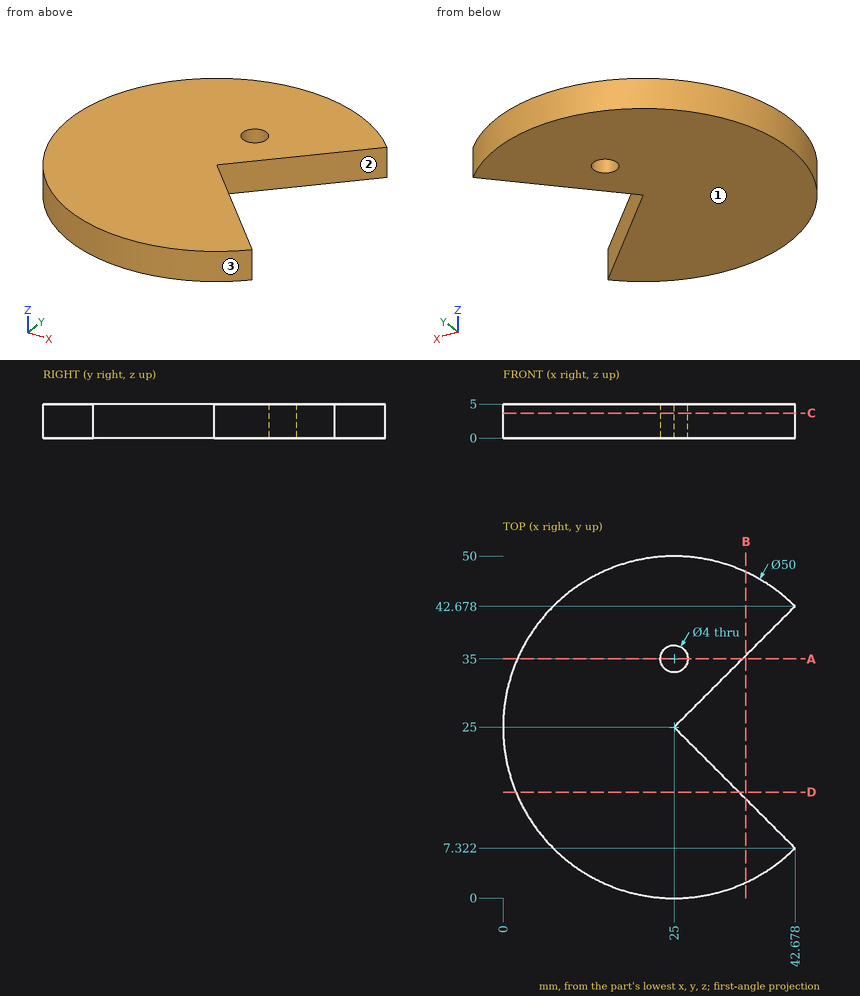
Geometry: see drawing. Coordinates: mm, zero at the bounding-box minimum. Coordinates: 2 decimals unless noted, no trailing zeros. Loops run counter-clockwise (first coordinate to the right, second up) from the corner with the lowest first, then second, coordinate; pieces in that order, holes last. Notation, with made-up numbers: (75, -26.75) - (128, -26.75) arc R13 ccw to (128, -21.75) - close; hole circle Ø11 at (31, 41.25). An arc over 180 degrees is marked (long way). Answer in a Markdown table with one row per item.
(1) Cut plane D-D on y = 15.5. Output: boundary loops of the cut face in (x, z) (1 decimal).
Model answer:
| item | result |
|---|---|
| outline | (1.9, 0) - (34.5, 0) - (34.5, 5) - (1.9, 5) - close |
(2) Cut plane B-B on x = 35.5. Output: boundary loops of the cut face in (y, z), plus the area to 3 significant figures.
Model answer:
| item | result |
|---|---|
| outline | (2.31, 0) - (14.5, 0) - (14.5, 5) - (2.31, 5) - close; (35.5, 0) - (47.69, 0) - (47.69, 5) - (35.5, 5) - close |
| area | 122 mm² |
(3) Material intervals for L1, parallel to Y at x = 33, z = 4.3 (1 decimal); L2, parallel to Y at x = 29, z = 1.85; L3, parallel to Y at x = 13, z = 4.3, sorted ascending. Write a range as from..to.
Model answer:
| item | result |
|---|---|
| L1 | y = 1.3..17, 33..48.7 |
| L2 | y = 0.32..21, 29..49.68 |
| L3 | y = 3.07..46.93 |
(4) Cut plane C-C on z = 3.65. Output: boundary loops of the cut face in (x, y).
Model answer:
| item | result |
|---|---|
| outline | (25, 25) - (42.68, 42.68) arc R25 ccw (long way) to (42.68, 7.32) - close; hole circle Ø4 at (25, 35) |
(5) Mould query, pull axis Y, two halves, no side actions, for the marked faces 1, 2 and 3. Classes: pulls with the +Y half, pulls with the -Y half, needs draft (parallel to the pull), parting line crosses it, or undercut.
Model answer:
| item | result |
|---|---|
| face 1 | needs draft |
| face 2 | undercut |
| face 3 | parting line crosses it |
(6) Pin query (flat end, axial travel): P1, Ø12, axis at x = 33, y = 18, coming from the +Z side; P2, Ø3, axis at x = 18, z = 2, coming from the -Y side. Return the tip coordinate at first contact, or that it passes through.
Model answer:
| item | result |
|---|---|
| P1 | stops at z = 5 |
| P2 | stops at y = 0.61 |
(7) Cut plane A-A on y = 35. Output: boundary loops of the cut face in (x, z), plus the area to 3 significant figures.
Model answer:
| item | result |
|---|---|
| outline | (2.09, 0) - (23, 0) - (23, 5) - (2.09, 5) - close; (27, 0) - (35, 0) - (35, 5) - (27, 5) - close |
| area | 145 mm² |
